from build123d import *

# Parameters (mm, degrees)
CROQUIS1_W              = 64
CROQUIS1_H              = 64
SALIENTE_EXTRUIR1_DEPTH = 60
CROQUIS2_W              = 70
CROQUIS2_H              = 70
CROQUIS2_W_2            = 64
CROQUIS2_H_2            = 64
SALIENTE_EXTRUIR2_DEPTH = 64
CORTAR_EXTRUIR1_DEPTH   = 21
CROQUIS5_R              = 1.1
CORTAR_EXTRUIR2_DEPTH   = 10
CORTAR_EXTRUIR3_REACH   = 30
CROQUIS10_R             = 4.5
CROQUIS11_W             = 70
CROQUIS11_H             = 70
CORTAR_EXTRUIR4_DEPTH   = 30
CROQUIS12_W             = 23
CROQUIS12_H             = 12.2
CORTAR_EXTRUIR5_DEPTH   = 21
CORTAR_EXTRUIR6_REACH   = 30
CROQUIS13_R             = 4.5
CROQUIS14_R             = 1.1
CORTAR_EXTRUIR7_DEPTH   = 10
CROQUIS15_R             = 3.7
CORTAR_EXTRUIR8_DEPTH   = 10
CROQUIS16_W             = 64
CROQUIS16_H             = 64
CORTAR_EXTRUIR9_DEPTH   = 5
CROQUIS17_W             = 12.5
CROQUIS17_H             = 12.998685397
CORTAR_EXTRUIR10_DEPTH  = 5
CORTAR_EXTRUIR11_REACH  = 72
CROQUIS18_W             = 70
CROQUIS18_H             = 9
CROQUIS18_H_2           = 5.000169364
CORTAR_EXTRUIR13_DEPTH  = 5
CORTAR_EXTRUIR16_REACH  = 5.001
CROQUIS23_W             = 3.1
CROQUIS23_H             = 12.5
CORTAR_EXTRUIR17_REACH  = 5
CROQUIS22_W             = 3.1
CROQUIS22_H             = 12.2


with BuildPart() as part:
    # Croquis1 → Saliente-Extruir1 (new body)
    with BuildSketch(Plane(origin=(0, 0, 0), x_dir=(1, 0, 0), z_dir=(0, 1, 0))):
        Rectangle(CROQUIS1_W, CROQUIS1_H)
    extrude(amount=SALIENTE_EXTRUIR1_DEPTH)

    # Croquis2 → Saliente-Extruir2 (add)
    with BuildSketch(Plane(origin=(0, 0, 0), x_dir=(1, 0, 0), z_dir=(0, 1, 0))):
        Rectangle(CROQUIS2_W, CROQUIS2_H)
        Rectangle(CROQUIS2_W_2, CROQUIS2_H_2, mode=Mode.SUBTRACT)
    extrude(amount=SALIENTE_EXTRUIR2_DEPTH)

    # Croquis4 → Cortar-Extruir1 (cut)
    with BuildSketch(Plane(origin=(0, 60, 0), x_dir=(1, 0, 0), z_dir=(0, 1, 0))):
        Polygon((-7, 6), (-7, -6), (-7, -6.25), (16, -6.25), (16, -6), (16, 6), (16, 6.25), (-7, 6.25), align=None)
    extrude(amount=-CORTAR_EXTRUIR1_DEPTH, mode=Mode.SUBTRACT)

    # Croquis5 → Cortar-Extruir2 (cut)
    with BuildSketch(Plane(origin=(0, 60, 0), x_dir=(1, 0, 0), z_dir=(0, 1, 0))):
        with Locations((19, 0)):
            Circle(CROQUIS5_R)
        with Locations((-9, 0)):
            Circle(CROQUIS5_R)
    extrude(amount=-CORTAR_EXTRUIR2_DEPTH, mode=Mode.SUBTRACT)

    # Croquis10 → Cortar-Extruir3 (cut, up to next)
    with BuildSketch(Plane(origin=(-7, 0, 0), x_dir=(0, 0, -1), z_dir=(1, 0, 0)), mode=Mode.PRIVATE) as cortar_extruir3_sk1:
        with Locations((0, 44)):
            Circle(CROQUIS10_R)
    cortar_extruir3_tool1 = extrude(cortar_extruir3_sk1.sketch, amount=-CORTAR_EXTRUIR3_REACH, mode=Mode.PRIVATE) & part.part
    add(cortar_extruir3_tool1.solids().sort_by_distance((-7, 44, 0))[0], mode=Mode.SUBTRACT)

    # Croquis11 → Cortar-Extruir4 (cut)
    with BuildSketch(Plane.XZ):
        Rectangle(CROQUIS11_W, CROQUIS11_H)
    extrude(amount=-CORTAR_EXTRUIR4_DEPTH, mode=Mode.SUBTRACT)

    # Croquis12 → Cortar-Extruir5 (cut)
    with BuildSketch(Plane.XZ.offset(-30)):
        with Locations((4.5, 22.1)):
            Rectangle(CROQUIS12_W, CROQUIS12_H)
    extrude(amount=-CORTAR_EXTRUIR5_DEPTH, mode=Mode.SUBTRACT)

    # Croquis13 → Cortar-Extruir6 (cut, up to next)
    with BuildSketch(Plane(origin=(-7, 0, 0), x_dir=(0, 0, -1), z_dir=(1, 0, 0)), mode=Mode.PRIVATE) as cortar_extruir6_sk1:
        with Locations((-22.1, 46)):
            Circle(CROQUIS13_R)
    cortar_extruir6_tool1 = extrude(cortar_extruir6_sk1.sketch, amount=-CORTAR_EXTRUIR6_REACH, mode=Mode.PRIVATE) & part.part
    add(cortar_extruir6_tool1.solids().sort_by_distance((-7, 46, 22.1))[0], mode=Mode.SUBTRACT)

    # Croquis14 → Cortar-Extruir7 (cut)
    with BuildSketch(Plane.XZ.offset(-30)):
        with Locations((19, 22.1)):
            Circle(CROQUIS14_R)
        with Locations((-9, 22.1)):
            Circle(CROQUIS14_R)
    extrude(amount=-CORTAR_EXTRUIR7_DEPTH, mode=Mode.SUBTRACT)

    # Croquis15 → Cortar-Extruir8 (cut)
    with BuildSketch(Plane.XZ.offset(-30)):
        with Locations((0, -22.1)):
            Circle(CROQUIS15_R)
    extrude(amount=-CORTAR_EXTRUIR8_DEPTH, mode=Mode.SUBTRACT)

    # Croquis16 → Cortar-Extruir9 (cut)
    with BuildSketch(Plane(origin=(0, 60, 0), x_dir=(1, 0, 0), z_dir=(0, 1, 0))):
        Rectangle(CROQUIS16_W, CROQUIS16_H)
    extrude(amount=-CORTAR_EXTRUIR9_DEPTH, mode=Mode.SUBTRACT)

    # Croquis17 → Cortar-Extruir10 (cut)
    with BuildSketch(Plane(origin=(-7, 0, 0), x_dir=(0, 0, -1), z_dir=(1, 0, 0))):
        with Locations((0, 45.499342699)):
            Rectangle(CROQUIS17_W, CROQUIS17_H)
    extrude(amount=-CORTAR_EXTRUIR10_DEPTH, mode=Mode.SUBTRACT)

    # Croquis18 → Cortar-Extruir11 (cut, up to next)
    with BuildSketch(Plane(origin=(35, 0, 0), x_dir=(0, 0, -1), z_dir=(1, 0, 0)), mode=Mode.PRIVATE) as cortar_extruir11_sk1:
        with Locations((0, 59.5)):
            Rectangle(CROQUIS18_W, CROQUIS18_H)
    cortar_extruir11_tool1 = extrude(cortar_extruir11_sk1.sketch, amount=-CORTAR_EXTRUIR11_REACH, mode=Mode.PRIVATE) & part.part
    add(cortar_extruir11_tool1.solids().sort_by_distance((35, 59.5, 0))[0], mode=Mode.SUBTRACT)
    # Croquis18 → Cortar-Extruir11 (cut, up to next)
    with BuildSketch(Plane(origin=(35, 0, 0), x_dir=(0, 0, -1), z_dir=(1, 0, 0)), mode=Mode.PRIVATE) as cortar_extruir11_sk2:
        with Locations((0, 32.500084682)):
            Rectangle(CROQUIS18_W, CROQUIS18_H_2)
    cortar_extruir11_tool2 = extrude(cortar_extruir11_sk2.sketch, amount=-CORTAR_EXTRUIR11_REACH, mode=Mode.PRIVATE) & part.part
    add(cortar_extruir11_tool2.solids().sort_by_distance((35, 32.500085, 0))[0], mode=Mode.SUBTRACT)

    # Croquis19 → Cortar-Extruir13 (cut)
    with BuildSketch(Plane(origin=(-7, 0, 0), x_dir=(0, 0, -1), z_dir=(1, 0, 0))):
        Polygon((-16, 51), (-28.2, 51), (-28.2, 38.000169364), (-22.1, 38.000169364), (-16, 38.000169364), align=None)
    extrude(amount=-CORTAR_EXTRUIR13_DEPTH, mode=Mode.SUBTRACT)

    # Croquis23 → Cortar-Extruir16 (cut, up to next)
    with BuildSketch(Plane.XZ.offset(-51.998685397), mode=Mode.PRIVATE) as cortar_extruir16_sk1:
        with Locations((-8.55, 0)):
            Rectangle(CROQUIS23_W, CROQUIS23_H)
    cortar_extruir16_tool1 = extrude(cortar_extruir16_sk1.sketch, amount=-CORTAR_EXTRUIR16_REACH, mode=Mode.PRIVATE) & part.part
    add(cortar_extruir16_tool1.solids().sort_by_distance((-8.55, 51.998685, 0))[0], mode=Mode.SUBTRACT)

    # Croquis22 → Cortar-Extruir17 (cut, up to next)
    with BuildSketch(Plane(origin=(0, 38.000169364, 0), x_dir=(1, 0, 0), z_dir=(0, 1, 0)), mode=Mode.PRIVATE) as cortar_extruir17_sk1:
        with Locations((-8.55, -22.1)):
            Rectangle(CROQUIS22_W, CROQUIS22_H)
    cortar_extruir17_tool1 = extrude(cortar_extruir17_sk1.sketch, amount=-CORTAR_EXTRUIR17_REACH, mode=Mode.PRIVATE) & part.part
    add(cortar_extruir17_tool1.solids().sort_by_distance((-8.55, 38.000169, 22.1))[0], mode=Mode.SUBTRACT)


solid = part.part
Can you work these out from the model? Positions are in its coordinate system, mm. A direction names the side the tool comes from. Give positions to 0.01 mm unless a question says otherwise; leave off trailing zeros. Write each loop counter-clockwise with the first axis right and the second up, starting at its lowest first coordinate (ties: lowest second). Pieces come first, ordered by that corner, then holes. Notation, with made-up numbers: M 37,21 L 83,21 A32 ccw 83,56 Z; hole C 70,74 d6. An arc over 180 degrees is marked long. Answer in a Markdown table with one row per item. Add a question column.
Item 1: We'd pull the mould along Y, two halves only. Please class faces 5 (the flat face through (-35, 49, 0)), 6 (the cylindrical face through (-23.34, 41.61, 23.08)), 7 (the flat face through (0, 35, 0)), 8 (the flat face through (19, 50, 0)): released by +Y, released by -Y, zero draft, split by the parting line, or undercut.
Item 2: Imagine slicing it at B-B, the plane x = 6. Write out the boundary of the cut face in (y, z).
Item 3: For pin 1 Ø6 at (x, z) = (1.5, 23.5) entering from -Y; pin 2 Ø6 at (x, z) = (-0.5, -3) entering from +Y; pin 3 Ø1.8 at (x, z) = (19, 22) entering from -Y, each with a flat end and sliding along its axis, tell me the tip position at first contact or that it passes through.
Item 4: Imagine slicing it at A-A, the plane z = 22.1. Write out the boundary of the cut face in (x, y), plus the area to 3 significant figures.
Item 5: On a 3-axis mill with a long thin cutter (end or side, diameter ignored), from which of +Z, -Z, +X, -X, +Y, -Y can I reach the whole of each face in a straight line? I mean faces 1 (the flat face through (-11, 51.999, 0)), 2 (the flat face through (-10.1, 37, 22)), 3 (the flat face through (-10.1, 53, 0)), 4 (the cylindrical face through (-23.34, 39.61, 0.98)). Say none if no direction works.
Item 6: Imagine slicing it at C-C, the plane x = -17. Write out the boundary of the cut face in (y, z), plus the area to 3 significant figures.
Item 7: Imagine slicing it at D-D, the plane z = 0. Write out the boundary of the cut face in (x, y), plus the area to 3 significant figures.
Item 8: Please list where these lines run through material, in increasing order: L1, parallel to X at y = 42.75, z = 6; L2, parallel to Z at x = 10, y = 52.5; L3, parallel to X at y = 52.25, z = 3.5.
Evaluation:
| question | item | result |
|---|---|---|
| 1 | face 5 | zero draft |
| 1 | face 6 | undercut |
| 1 | face 7 | released by -Y |
| 1 | face 8 | released by +Y |
| 2 | outline | M 35,-35 L 55,-35 L 55,-6.25 L 39,-6.25 L 39,6.25 L 55,6.25 L 55,35 L 35,35 L 35,28.2 L 51,28.2 L 51,16 L 35,16 Z |
| 3 | pin 1 | stops at y = 51 |
| 3 | pin 2 | stops at y = 39 |
| 3 | pin 3 | stops at y = 40 |
| 4 | outline | M -35,35 L -10.1,35 L -10.1,38 L -12,38 L -12,41.5 L -35,41.5 Z; M -35,50.5 L -12,50.5 L -12,51 L 16,51 L 16,35 L 17.9,35 L 17.9,40 L 20.1,40 L 20.1,35 L 35,35 L 35,55 L -35,55 Z |
| 4 | area | 740 mm² |
| 5 | face 1 | none |
| 5 | face 2 | -Y |
| 5 | face 3 | +Y |
| 5 | face 4 | -X |
| 6 | outline | M 35,-35 L 55,-35 L 55,35 L 35,35 Z; hole C 44,0 d9; hole C 46,22.1 d9 |
| 6 | area | 1,270 mm² |
| 7 | outline | M -35,35 L 35,35 L 35,55 L 20.1,55 L 20.1,50 L 17.9,50 L 17.9,55 L 16,55 L 16,39 L -12,39 L -12,39.5 L -35,39.5 Z; M -35,48.5 L -12,48.5 L -12,52 L -10.1,52 L -10.1,55 L -35,55 Z |
| 7 | area | 740 mm² |
| 8 | L1 | x = -35 to -12, 16 to 35 |
| 8 | L2 | z = -35 to -6.25, 6.25 to 35 |
| 8 | L3 | x = -35 to -10.1, 16 to 35 |
